Could you check a few things on this model? Use its own coordinates, in mm. Face numbers are marked on the shaded views. A direction names the side the tool comes from. Give positions to 0.01 mm unless a question says otherwise; leave off trailing zeros. Order: outer loops, then holes, each group sorted by start corner. A loop starts at its lowest first (then second) coordinate and runs counter-clockwise, first axis right, second up.
from build123d import *

# Parameters (mm, degrees)
PAD_DEPTH       = 20
SKETCH002_R     = 15
POCKET001_DEPTH = 20
SKETCH003_R     = 15
POCKET002_DEPTH = 20
SKETCH_R        = 45
PAD001_DEPTH    = 90
SKETCH004_R     = 40
POCKET_DEPTH    = 25
SKETCH005_R     = 30
POCKET003_DEPTH = 110


with BuildPart() as part:
    # Sketch001 → Pad (new body)
    with BuildSketch(Plane.XZ):
        with BuildLine():
            Line((20.821842, 56.271226), (99.135441, 28.576132))
            ThreePointArc((99.258042, -28.53666), (120.002757, 0.064399), (99.135441, 28.576132))
            Line((99.258042, -28.53666), (25.71069, -54.21218))
            ThreePointArc((-18.562526, -57.056399), (3.846616, -59.876569), (25.71069, -54.21218))
            Line((-18.562526, -57.056399), (-99.28142, -28.602251))
            ThreePointArc((-99.262461, 28.63761), (-120.277525, 0.024636), (-99.28142, -28.602251))
            Line((-18.539501, 57.063884), (-99.262461, 28.63761))
            ThreePointArc((20.821842, 56.271226), (1.208034, 59.987838), (-18.539501, 57.063884))
        make_face()
    extrude(amount=PAD_DEPTH)

    # Sketch002 → Pocket001 (cut)
    with BuildSketch(Plane(origin=(0, 0, 0), x_dir=(1, 0, 0), z_dir=(0, 1, 0))):
        with Locations((-90, 0)):
            Circle(SKETCH002_R)
    extrude(amount=-POCKET001_DEPTH, mode=Mode.SUBTRACT)

    # Sketch003 (on Face4 of Pocket001) → Pocket002 (cut)
    with BuildSketch(Plane(origin=(0, 0, 0), x_dir=(1, 0, 0), z_dir=(0, 1, 0))):
        with Locations((90, 0)):
            Circle(SKETCH003_R)
    extrude(amount=-POCKET002_DEPTH, mode=Mode.SUBTRACT)

    # Sketch (on Face9 of Pad) → Pad001 (join)
    with BuildSketch(Plane(origin=(0, 0, 0), x_dir=(1, 0, 0), z_dir=(0, 1, 0))):
        Circle(SKETCH_R)
    extrude(amount=PAD001_DEPTH)

    # Sketch004 (on Face14 of Pad001) → Pocket (cut)
    with BuildSketch(Plane(origin=(0, 90, 0), x_dir=(1, 0, 0), z_dir=(0, 1, 0))):
        with Locations((0.371243, -0.842497)):
            Circle(SKETCH004_R)
    extrude(amount=-POCKET_DEPTH, mode=Mode.SUBTRACT)

    # Sketch005 (on Face16 of Pocket) → Pocket003 (cut)
    with BuildSketch(Plane(origin=(0, 65, 0), x_dir=(1, 0, 0), z_dir=(0, 1, 0))):
        Circle(SKETCH005_R)
    extrude(amount=-POCKET003_DEPTH, mode=Mode.SUBTRACT)


solid = part.part
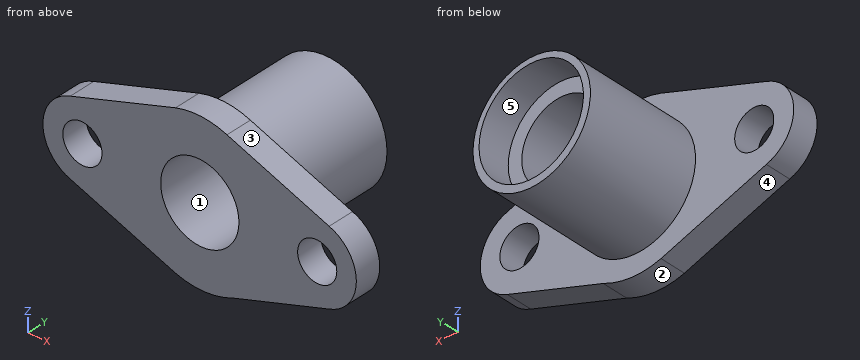
Item 1: For the marked faces 4 and 5, which set-ups out of +Z, -Z, +X, -X, +Y, -Y let a thin tool reach every point of the face, with its end or its side?
Findings:
face 4: -Z, -X, +Y, -Y
face 5: +Y
Item 2: We'd pull the mould along Z, two halves only. Please class the marked faces 1, 2 and 3: +Z half, -Z half, draft (parallel to the pull), parting line (faces both ways), or undercut.
Findings:
face 1: undercut
face 2: -Z half
face 3: +Z half
Item 3: Imagine slicing it at B-B on x = -4. List the corners of the cut face in (y, z) for me.
Findings:
outline: (-20, -59.87) - (0, -59.87) - (0, -44.82) - (90, -44.82) - (90, -38.92) - (65, -38.92) - (65, -29.73) - (-20, -29.73) - close; (-20, 29.73) - (65, 29.73) - (65, 40.6) - (90, 40.6) - (90, 44.82) - (0, 44.82) - (0, 59.87) - (-20, 59.87) - close
Item 4: Imagine slicing it at D-D on z = 19.5. List the corners of the cut face in (x, y) for me.
Findings:
outline: (-113.09, -20) - (-22.8, -20) - (-22.8, 65) - (-35.01, 65) - (-35.01, 90) - (-40.56, 90) - (-40.56, 0) - (-113.09, 0) - close; (22.8, -20) - (112.8, -20) - (112.8, 0) - (40.56, 0) - (40.56, 90) - (35.75, 90) - (35.75, 65) - (22.8, 65) - close
Item 5: Imagine slicing it at C-C on z = 7. List the corners of the cut face in (x, y) for me.
Findings:
outline: (-119.45, -20) - (-103.27, -20) - (-103.27, 0) - (-119.45, 0) - close; (-76.73, -20) - (-29.17, -20) - (-29.17, 65) - (-39.15, 65) - (-39.15, 90) - (-44.45, 90) - (-44.45, 0) - (-76.73, 0) - close; (29.17, -20) - (76.73, -20) - (76.73, 0) - (44.45, 0) - (44.45, 90) - (39.89, 90) - (39.89, 65) - (29.17, 65) - close; (103.27, -20) - (119.17, -20) - (119.17, 0) - (103.27, 0) - close
Item 6: For pin 1 (2 mm diameter, centred on x = 1.5, y = 0.5, fed in from +Z); pin 2 (1 mm diameter, centred on y = 41.5, z = 20, fed in from +X); pin 3 (4 mm diameter, centred on x = -31, y = 12.5, fed in from -Z); pin 4 (10 mm diameter, centred on x = 0.5, y = -5.5, fed in from -Z), each with a flat end and sliding along its axis, tell me the tip position at first contact or that it passes through.
Findings:
pin 1: stops at z = 60
pin 2: stops at x = 40.56
pin 3: stops at z = -34.41
pin 4: stops at z = -60
Item 7: Please list where these lines run through material, in increasing order: line 1 along X through (y, z) = (-5.75, 0); line 2 along Z through (x, y) = (0, 5); line 3 along X through (y, z) = (46.5, -1.5) (3 decimals).
Findings:
line 1: x = -120.28 to -105, -75 to -30, 30 to 75, 105 to 120
line 2: z = -45 to -30, 30 to 45
line 3: x = -44.975 to -29.962, 29.962 to 44.975
Item 8: Imagine slicing it at A-A on y = -5.5. List the corners of the cut face in (x, z) for me, then the cut area to 3 significant figures.
Findings:
outline: (-99.28, -28.6) - (-18.56, -57.06) arc R60 ccw to (25.71, -54.21) - (99.26, -28.54) arc R30 ccw to (99.14, 28.58) - (20.82, 56.27) arc R60 ccw to (-18.54, 57.06) - (-99.26, 28.64) arc R30 ccw to start; hole circle Ø30 at (-90, 0); hole circle Ø60 at (0, 0); hole circle Ø30 at (90, 0)
area: 15,700 mm2
